from build123d import *
from OCP.BRepFilletAPI import BRepFilletAPI_MakeChamfer

# Parameters (mm, degrees)
SKETCH1_W           = 48.514
SKETCH1_H           = 54.102
BOSS_EXTRUDE1_DEPTH = 17.1196
SKETCH3_W           = 48.514
SKETCH3_H           = 32.258
BOSS_EXTRUDE3_DEPTH = 19.304
CHAMFER1_SIZE       = 6.985
CHAMFER1_SIZE2      = 9.525
CHAMFER3_SIZE       = 2.159
CHAMFER4_SIZE       = 1.143
CHAMFER4_SIZE2      = 1.183611149
SKETCH4_R           = 3.175
CUT_EXTRUDE1_DEPTH  = 5.08
LPATTERN1_COUNT     = 2
LPATTERN1_PITCH     = 14.3002
LPATTERN1_COL_COUNT = 2
LPATTERN1_COL_PITCH = 14.3002


with BuildPart() as part:
    # Sketch1 → Boss-Extrude1 (new body)
    with BuildSketch(Plane(origin=(0, 0, 0), x_dir=(1, 0, 0), z_dir=(0, 1, 0))):
        with Locations((24.257, -27.051)):
            Rectangle(SKETCH1_W, SKETCH1_H)
    extrude(amount=BOSS_EXTRUDE1_DEPTH)

    # Sketch3 → Boss-Extrude3 (add)
    with BuildSketch(Plane(origin=(0, 17.1196, 0), x_dir=(1, 0, 0), z_dir=(0, 1, 0))):
        with Locations((24.257, -25.781)):
            Rectangle(SKETCH3_W, SKETCH3_H)
    extrude(amount=BOSS_EXTRUDE3_DEPTH)

    # Chamfer1: one chamfer whose edges measure the first distance from different faces: ONE call of the kernel's chamfer builder (chamfer() names one face for all edges)
    chamfer1_edges_1 = [part.edges().sort_by_distance(p)[0] for p in [
        (0, 36.4236, 25.781),
    ]]
    chamfer1_side_1 = [part.faces().sort_by_distance(p)[0] for p in [
        (0, 15.881477327, 26.540422781),
    ]]
    chamfer1_edges_2 = [part.edges().sort_by_distance(p)[0] for p in [
        (48.514, 36.4236, 25.781),
    ]]
    chamfer1_side_2 = [part.faces().sort_by_distance(p)[0] for p in [
        (48.514, 15.881477327, 26.540422781),
    ]]
    chamfer1 = BRepFilletAPI_MakeChamfer(part.part.solid().wrapped)
    for e in chamfer1_edges_1:
        chamfer1.Add(CHAMFER1_SIZE, CHAMFER1_SIZE2, e.wrapped, chamfer1_side_1[0].wrapped)  # the first distance lies on this face
    for e in chamfer1_edges_2:
        chamfer1.Add(CHAMFER1_SIZE, CHAMFER1_SIZE2, e.wrapped, chamfer1_side_2[0].wrapped)  # the first distance lies on this face
    add(Compound.cast(chamfer1.Shape()), mode=Mode.REPLACE)

    # Chamfer3
    chamfer3_edges = [part.edges().sort_by_distance(p)[0] for p in [
        (0, 8.5598, 0),
        (48.514, 8.5598, 0),
        (48.514, 8.5598, 54.102),
        (0, 8.5598, 54.102),
    ]]
    chamfer(chamfer3_edges, length=CHAMFER3_SIZE)

    # Chamfer4: one chamfer whose edges measure the first distance from different faces: ONE call of the kernel's chamfer builder (chamfer() names one face for all edges)
    chamfer4_edges_1 = [part.edges().sort_by_distance(p)[0] for p in [
        (0, 17.1196, 46.9265),
        (0, 17.1196, 5.9055),
    ]]
    chamfer4_side_1 = [part.faces().sort_by_distance(p)[0] for p in [
        (0, 13.24043998, 26.647148406),
    ]]
    chamfer4_edges_2 = [part.edges().sort_by_distance(p)[0] for p in [
        (48.514, 17.1196, 5.9055),
        (48.514, 17.1196, 46.9265),
    ]]
    chamfer4_side_2 = [part.faces().sort_by_distance(p)[0] for p in [
        (48.514, 13.24043998, 26.647148406),
    ]]
    chamfer4_edges_3 = [part.edges().sort_by_distance(p)[0] for p in [
        (24.257, 17.1196, 0),
    ]]
    chamfer4_side_3 = [part.faces().sort_by_distance(p)[0] for p in [
        (24.257, 8.5598, 0),
    ]]
    chamfer4_edges_4 = [part.edges().sort_by_distance(p)[0] for p in [
        (47.4345, 17.1196, 1.0795),
    ]]
    chamfer4_side_4 = [part.faces().sort_by_distance(p)[0] for p in [
        (47.4345, 8.5598, 1.0795),
    ]]
    chamfer4_edges_5 = [part.edges().sort_by_distance(p)[0] for p in [
        (1.0795, 17.1196, 1.0795),
    ]]
    chamfer4_side_5 = [part.faces().sort_by_distance(p)[0] for p in [
        (1.0795, 8.5598, 1.0795),
    ]]
    chamfer4_edges_6 = [part.edges().sort_by_distance(p)[0] for p in [
        (24.257, 17.1196, 54.102),
    ]]
    chamfer4_side_6 = [part.faces().sort_by_distance(p)[0] for p in [
        (24.257, 8.5598, 54.102),
    ]]
    chamfer4_edges_7 = [part.edges().sort_by_distance(p)[0] for p in [
        (1.0795, 17.1196, 53.0225),
    ]]
    chamfer4_side_7 = [part.faces().sort_by_distance(p)[0] for p in [
        (1.0795, 8.5598, 53.0225),
    ]]
    chamfer4_edges_8 = [part.edges().sort_by_distance(p)[0] for p in [
        (47.4345, 17.1196, 53.0225),
    ]]
    chamfer4_side_8 = [part.faces().sort_by_distance(p)[0] for p in [
        (47.4345, 8.5598, 53.0225),
    ]]
    chamfer4 = BRepFilletAPI_MakeChamfer(part.part.solid().wrapped)
    for e in chamfer4_edges_1:
        chamfer4.Add(CHAMFER4_SIZE, CHAMFER4_SIZE2, e.wrapped, chamfer4_side_1[0].wrapped)  # the first distance lies on this face
    for e in chamfer4_edges_2:
        chamfer4.Add(CHAMFER4_SIZE, CHAMFER4_SIZE2, e.wrapped, chamfer4_side_2[0].wrapped)  # the first distance lies on this face
    for e in chamfer4_edges_3:
        chamfer4.Add(CHAMFER4_SIZE, CHAMFER4_SIZE2, e.wrapped, chamfer4_side_3[0].wrapped)  # the first distance lies on this face
    for e in chamfer4_edges_4:
        chamfer4.Add(CHAMFER4_SIZE, CHAMFER4_SIZE2, e.wrapped, chamfer4_side_4[0].wrapped)  # the first distance lies on this face
    for e in chamfer4_edges_5:
        chamfer4.Add(CHAMFER4_SIZE, CHAMFER4_SIZE2, e.wrapped, chamfer4_side_5[0].wrapped)  # the first distance lies on this face
    for e in chamfer4_edges_6:
        chamfer4.Add(CHAMFER4_SIZE, CHAMFER4_SIZE2, e.wrapped, chamfer4_side_6[0].wrapped)  # the first distance lies on this face
    for e in chamfer4_edges_7:
        chamfer4.Add(CHAMFER4_SIZE, CHAMFER4_SIZE2, e.wrapped, chamfer4_side_7[0].wrapped)  # the first distance lies on this face
    for e in chamfer4_edges_8:
        chamfer4.Add(CHAMFER4_SIZE, CHAMFER4_SIZE2, e.wrapped, chamfer4_side_8[0].wrapped)  # the first distance lies on this face
    add(Compound.cast(chamfer4.Shape()), mode=Mode.REPLACE)

    # Sketch4 → Cut-Extrude1 (cut)
    with BuildSketch(Plane(origin=(0, 17.1196, 0), x_dir=(1, 0, 0), z_dir=(0, 1, 0))):
        with Locations(Location((24.257, -46.695388851, 0), (0, 0, 270))):
            Circle(SKETCH4_R)
    cut_extrude1 = extrude(amount=-CUT_EXTRUDE1_DEPTH, mode=Mode.SUBTRACT)

    # LPattern1: Cut-Extrude1 ×2
    with Locations(*[(i * LPATTERN1_PITCH, 0, 0) for i in range(1, LPATTERN1_COUNT)]):
        add(cut_extrude1, mode=Mode.SUBTRACT)

    # LPattern1 col: Cut-Extrude1 ×2
    with Locations(*[(-i * LPATTERN1_COL_PITCH, 0, 0) for i in range(1, LPATTERN1_COL_COUNT)]):
        add(cut_extrude1, mode=Mode.SUBTRACT)


solid = part.part
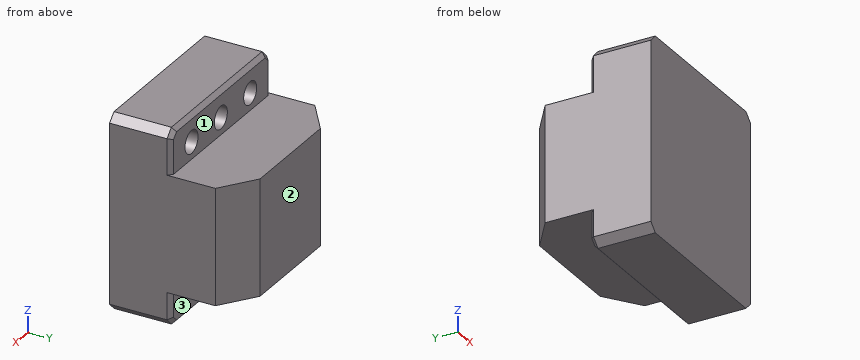
Verification items for the finished model (mm, model axes). Face numbers are marked on the shaded views. A direction names the side the tool comes from. Give positions to 0.01 mm unless a question says otherwise; leave off trailing zeros. Loops run counter-clockwise (first coordinate to the right, second up) from the corner with the lowest first, then second, coordinate; pieces in that order, holes last.
1. Go/stop test with flat-tipped pins: P1, Ø3, axis at x = 9.5, z = 45.5, coming from the +Y side; P2, Ø5, axis at x = 39.5, z = 47.5, coming from the +Y side; P3, Ø6, axis at x = 12.5, y = 29.5, coming from the -Z side. Record where each tip stops, or that it passes through.
Derived:
P1: stops at y = 12.04
P2: stops at y = 17.12
P3: stops at z = 9.65
2. Cross-section at A-A on x = 19. Record the cut outline in (y, z).
Derived:
outline: (0, 0) - (15.98, 0) - (17.12, 1.18) - (17.12, 9.65) - (36.42, 9.65) - (36.42, 41.91) - (17.12, 41.91) - (17.12, 52.92) - (15.98, 54.1) - (0, 54.1) - close
3. Cross-section at B-B on z = 26. Record the cut outline in (x, y) (3 decimals).
Derived:
outline: (0, 0) - (48.514, 0) - (48.514, 29.439) - (38.989, 36.424) - (9.525, 36.424) - (0, 29.439) - close
4. Tool access check on the marked faces 1, 2 and 3. Record the directions out of +Z, -Z, +X, -X, +Y, -Y that give a thin tool (end or side, any length) a straight path to the whole face; none if there is none.
Derived:
face 1: +Z, +X, -X, +Y
face 2: +Z, -Z, +X, -X, +Y
face 3: -Z, +X, -X, +Y
5. Material ranges on probe 1 along Z at (x, y) = (35.5, 23); probe 2 along Y at (x, z) = (24, 8.5); probe 3 along Z at (x, y) = (11.5, 14), recorded low to high.
Derived:
probe 1: z = 9.65 to 41.91
probe 2: y = 0 to 17.12
probe 3: z = 0 to 43.92, 49.47 to 54.1
6. Cross-section at C-C on y = 28. Record the cut outline in (x, z), and give its area (3 significant figures).
Derived:
outline: (0, 9.65) - (48.51, 9.65) - (48.51, 41.91) - (0, 41.91) - close
area: 1,560 mm2
7. Cross-section at D-D on x = 45. Record the cut outline in (y, z), and give its area (3 significant figures).
Derived:
outline: (0, 0) - (15.98, 0) - (17.12, 1.18) - (17.12, 9.65) - (32.02, 9.65) - (32.02, 41.91) - (17.12, 41.91) - (17.12, 52.92) - (15.98, 54.1) - (0, 54.1) - close
area: 1,410 mm2
